Read the model definition and answer for the solid it produces. Units are mm, in the model's axes. Coordinates: 2 decimals unless noted, no trailing zeros. Order: outer loops, then holes, each group sorted by start corner. A loop starts at its lowest first (then second) coordinate and runs counter-clockwise, first axis right, second up.
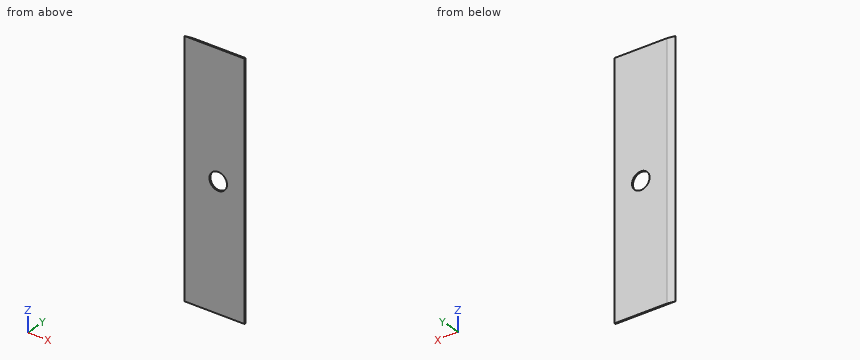
from build123d import *

# Parameters (mm, degrees)
BOSS_EXTRUDE1_DEPTH = 11.938
SKETCH3_R           = 0.8509
CUT_EXTRUDE1_DEPTH  = 0.127


with BuildPart() as part:
    # Sketch2 → Boss-Extrude1 (new, symmetric)
    with BuildSketch(Plane.XY):
        Polygon((0, 0), (5.08, 0), (5.08, 0.127), (0, 0.127), (-0.720252791, 0), align=None)
    extrude(amount=BOSS_EXTRUDE1_DEPTH, both=True)

    # Sketch3 → Cut-Extrude1 (cut)
    with BuildSketch(Plane(origin=(0, 0.127, 0), x_dir=(1, 0, 0), z_dir=(0, 1, 0))):
        with Locations(Location((2.54, 0, 0), (0, 0, 180))):
            Circle(SKETCH3_R)
    extrude(amount=-CUT_EXTRUDE1_DEPTH, mode=Mode.SUBTRACT)


solid = part.part
Q1. Each of these flat-tipped pins is pushed along its axis until it touches: P1, Ø1.5, axis at x = 2.54, z = 0, coming from the +Y side; P2, Ø3, axis at x = 1, z = -3.5, coming from the -Y side. Where does it stop, or does it pass through?
Q2. The part is cut by section A-A, the plane z = 0. Determine the outline of the cut face in (x, y).
Q3. A straight line is drawn through the part: L1, parallel to Z at x = 2.54, y = 0.05. Find the intervals that lie inside material, in ascending order.
Q4. The part is cut by section C-C, the plane z = -5.75. Determine the outline of the cut face in (x, y), then the cut area to 3 significant figures.
Q5. The part is cut by section B-B, the plane x = 2.54. Determine the outline of the cut face in (y, z), then the cut area to 3 significant figures.
Computed values:
1. P1: passes through
1. P2: stops at y = 0
2. outline: (-0.72, 0) - (1.69, 0) - (1.69, 0.13) - (0, 0.13) - close; (3.39, 0) - (5.08, 0) - (5.08, 0.13) - (3.39, 0.13) - close
3. L1: z = -11.94 to -0.85, 0.85 to 11.94
4. outline: (-0.72, 0) - (5.08, 0) - (5.08, 0.13) - (0, 0.13) - close
4. area: 0.691 mm2
5. outline: (0, -11.94) - (0.13, -11.94) - (0.13, -0.85) - (0, -0.85) - close; (0, 0.85) - (0.13, 0.85) - (0.13, 11.94) - (0, 11.94) - close
5. area: 2.82 mm2
